from build123d import *

# Parameters (mm, degrees)
SKETCH1_R           = 2.25
BOSS_EXTRUDE2_DEPTH = 5
BOSS_EXTRUDE3_DEPTH = 30
SKETCH4_W           = 140
SKETCH4_H           = 4
BOSS_EXTRUDE4_DEPTH = 30
CUT_EXTRUDE1_REACH  = 236.178
FILLET1_R           = 10


with BuildPart() as part:
    # Sketch1 → Boss-Extrude2 (new body)
    with BuildSketch(Plane(origin=(0, 0, 0), x_dir=(1, 0, 0), z_dir=(0, 1, 0))):
        with BuildLine():
            Line((-70, 90.5), (70, 90.5))
            ThreePointArc((70, 90.5), (84.142135624, 84.642135624), (90, 70.5))
            Line((90, 70.5), (90, -75.2))
            ThreePointArc((90, -75.2), (84.142135624, -89.342135624), (70, -95.2))
            Line((70, -95.2), (-70, -95.2))
            ThreePointArc((-70, -95.2), (-84.142135624, -89.342135624), (-90, -75.2))
            Line((-90, -75.2), (-90, 70.5))
            ThreePointArc((-90, 70.5), (-84.142135624, 84.642135624), (-70, 90.5))
        make_face()
        with Locations(Location((-70, 70, 0), (0, 0, 270))):
            Circle(SKETCH1_R, mode=Mode.SUBTRACT)
        with Locations(Location((70, 70, 0), (0, 0, 270))):
            Circle(SKETCH1_R, mode=Mode.SUBTRACT)
        with Locations(Location((-70, -70, 0), (0, 0, 270))):
            Circle(SKETCH1_R, mode=Mode.SUBTRACT)
        with Locations(Location((70, -70, 0), (0, 0, 270))):
            Circle(SKETCH1_R, mode=Mode.SUBTRACT)
        with BuildLine():
            Line((40, -60), (-40, -60))
            ThreePointArc((-40, -60), (-54.142135624, -54.142135624), (-60, -40))
            Line((-60, -40), (-60, 40))
            ThreePointArc((-60, 40), (-54.142135624, 54.142135624), (-40, 60))
            Line((-40, 60), (40, 60))
            ThreePointArc((40, 60), (54.142135624, 54.142135624), (60, 40))
            Line((60, 40), (60, -40))
            ThreePointArc((60, -40), (54.142135624, -54.142135624), (40, -60))
        make_face(mode=Mode.SUBTRACT)
    extrude(amount=BOSS_EXTRUDE2_DEPTH)

    # Sketch1<3> → Boss-Extrude3 (add)
    with BuildSketch(Plane(origin=(0, 0, 0), x_dir=(1, 0, 0), z_dir=(0, 1, 0))):
        with BuildLine():
            Line((-70, -95.2), (-70, -103.2))
            ThreePointArc((-70, -103.2), (-67.071067812, -110.271067812), (-60, -113.2))
            Line((-60, -113.2), (60, -113.2))
            ThreePointArc((60, -113.2), (67.071067812, -110.271067812), (70, -103.2))
            Line((70, -103.2), (70, -95.2))
            Line((70, -95.2), (-70, -95.2))
        make_face()
        with BuildLine():
            ThreePointArc((-70, 98.5), (-67.071067812, 105.571067812), (-60, 108.5))
            Line((-60, 108.5), (60, 108.5))
            ThreePointArc((60, 108.5), (67.071067812, 105.571067812), (70, 98.5))
            Line((70, 98.5), (70, 90.5))
            Line((70, 90.5), (-70, 90.5))
            Line((-70, 90.5), (-70, 98.5))
        make_face()
    extrude(amount=BOSS_EXTRUDE3_DEPTH)

    # Sketch4 → Boss-Extrude4 (add)
    with BuildSketch(Plane(origin=(0, 30, 0), x_dir=(1, 0, 0), z_dir=(0, 1, 0))):
        with Locations((0, 92.5)):
            Rectangle(SKETCH4_W, SKETCH4_H)
        with Locations((0, -97.2)):
            Rectangle(SKETCH4_W, SKETCH4_H)
    extrude(amount=BOSS_EXTRUDE4_DEPTH)

    # Cut-Extrude1: up to this face of the body (flat: up to its plane)
    cut_extrude1_end = Plane(part.part.faces().sort_by_distance((0, 45, -94.5))[0])
    # Sketch5 → Cut-Extrude1 (cut, up to the picked face)
    with BuildSketch(Plane.XY.offset(99.2), mode=Mode.PRIVATE) as cut_extrude1_sk1:
        with BuildLine():
            Line((-63.303955024, 52.25), (60.438343891, 52.25))
            ThreePointArc((60.438343891, 52.25), (62.688343891, 50), (60.438343891, 47.75))
            Line((60.438343891, 47.75), (-63.303955024, 47.75))
            ThreePointArc((-63.303955024, 47.75), (-65.553955024, 50), (-63.303955024, 52.25))
        make_face()
    cut_extrude1_tool1 = split(extrude(cut_extrude1_sk1.sketch, amount=-CUT_EXTRUDE1_REACH, mode=Mode.PRIVATE), bisect_by=cut_extrude1_end, keep=Keep.BOTH, mode=Mode.PRIVATE)
    add(cut_extrude1_tool1.solids().sort_by(Axis((-1.432806, 50, 99.2), (0, 0, -1)))[0], mode=Mode.SUBTRACT)

    # Fillet1
    # the kernel refuses this fillet: 10 mm, written as the material it adds along each edge
    with BuildSketch(Plane(origin=(70, 5, 95.2), x_dir=(0, 0, -1), z_dir=(-1, 0, 0)), Plane(origin=(-70, 5, -90.5), x_dir=(0, 0, 1), z_dir=(1, 0, 0))) as fillet1_piece_1:
        with BuildLine():
            CenterArc((FILLET1_R, -FILLET1_R), FILLET1_R, 90, 90)
            Line((0, -FILLET1_R), (0, 0))
            Line((0, 0), (FILLET1_R, 0))
        make_face()
    extrude(amount=140)


solid = part.part
Work out the finished part from the listing and answer in its coordinate system (mm). A direction names the side the tool comes from. Give positions to 0.01 mm unless a question says otherwise; leave off trailing zeros. Order: outer loops, then holes, each group sorted by start corner. A loop starts at its lowest first (then second) coordinate and runs counter-clockwise, first axis right, second up. Notation, with made-up numbers: (63, -30) -> (91, -30) arc R33 cw to (91, 6) -> close; hole circle Ø10 at (59.25, 34.25). An arc over 180 degrees is marked (long way). Answer as a JSON object with one key per item and string values. Group by question number.
1. Flat-ended cylindrical pins translate along their axes: pin 1 Ø1.2 at (x, z) = (10.5, -93.5) entering from -Y; pin 2 Ø4 at (x, z) = (-19.5, 68.5) entering from +Y; pin 3 Ø13.5 at (x, y) = (-14, 38.5) entering from -Z; pin 4 Ø3.5 at (x, z) = (-70, -70) entering from +Y. Find the tip coordinate at first contact, or state that the pin passes through.
2. Consider line 1 along X through (y, z) = (2.4, 70); line 2 along Z through (x, y) = (47.5, 46); line 3 along Z through (x, y) = (10.5, 15). Determine where each line is inside the solid, lowest interval first. Write a range as [from, to].
3. Section B-B on z = 54.5 is taken. Determine the outline of the cut face in (x, y), plus the area to 3 significant figures.
4. Section A-A on x = 12.5 is taken. Determine the outline of the cut face in (y, z), plus the area to 3 significant figures.
5. The mould has two halves that part along X. Classify faces 1 (the cylindrical face through (-83.986, 2.465, 89.497)), 2 (the cylindrical face through (83.986, 2.465, -84.797)), 3 (the cylindrical face through (-53.986, 2.465, 54.297)): released by +X, released by -X, zero draft, split by the parting line, or undercut.
6. Section D-D on z = 8.5 is taken. Determine the outline of the cut face in (x, y).
7. Section C-C on y = 9.5 is taken. Determine the outline of the cut face in (x, z).
8. A tool of negligible diameter and unlimited length cuts with its end or side. For faces 4 (the flat face through (-1, 45, 99.2)), 5 (the cylindrical face through (-0.98, 7.85, -87.49)), 6 (the flat face through (60, 2, -1)), 7 (the flat face through (1, 30, -102)), 8 (the cylindrical face through (66.99, 14.79, -105.65)), from which of +Z, -Z, +X, -X, +Y, -Y can it reach the whole face along a straight path? Write none if from no direction.
Result sheet:
{
 "1": {"pin 1": "stops at y = 0", "pin 2": "stops at y = 5", "pin 3": "stops at z = -94.5", "pin 4": "passes through"},
 "2": {"line 1": "x = [-90, -72.25], [-67.75, 67.75], [72.25, 90]", "line 2": "z = [-94.5, -90.5], [95.2, 99.2]", "line 3": "z = [-108.5, -90.5], [95.2, 113.2]"},
 "3": {"outline": "(-90, 0) -> (-53.77, 0) -> (-53.77, 5) -> (-90, 5) -> close; (53.77, 0) -> (90, 0) -> (90, 5) -> (53.77, 5) -> close", "area": "362 mm^2"},
 "4": {"outline": "(0, -108.5) -> (30, -108.5) -> (30, -94.5) -> (47.75, -94.5) -> (47.75, -90.5) -> (15, -90.5) arc R10 cw to (5, -80.5) -> (5, -60) -> (0, -60) -> close; (0, 60) -> (5, 60) -> (5, 85.2) arc R10 cw to (15, 95.2) -> (47.75, 95.2) -> (47.75, 99.2) -> (30, 99.2) -> (30, 113.2) -> (0, 113.2) -> close; (52.25, -94.5) -> (60, -94.5) -> (60, -90.5) -> (52.25, -90.5) -> close; (52.25, 95.2) -> (60, 95.2) -> (60, 99.2) -> (52.25, 99.2) -> close", "area": "1,660 mm^2"},
 "5": {"face 1": "released by -X", "face 2": "released by +X", "face 3": "undercut"},
 "6": {"outline": "(-90, 0) -> (-60, 0) -> (-60, 5) -> (-90, 5) -> close; (60, 0) -> (90, 0) -> (90, 5) -> (60, 5) -> close"},
 "7": {"outline": "(-70, -98.5) arc R10 ccw to (-60, -108.5) -> (60, -108.5) arc R10 ccw to (70, -98.5) -> (70, -88.85) -> (-70, -88.85) -> close; (-70, 93.55) -> (70, 93.55) -> (70, 103.2) arc R10 ccw to (60, 113.2) -> (-60, 113.2) arc R10 ccw to (-70, 103.2) -> close"},
 "8": {"face 4": "+Z, +X, -X, +Y", "face 5": "+X, -X, +Y", "face 6": "+Y, -Y", "face 7": "-Z, +X, -X, +Y", "face 8": "-Z, +X, +Y, -Y"}
}
